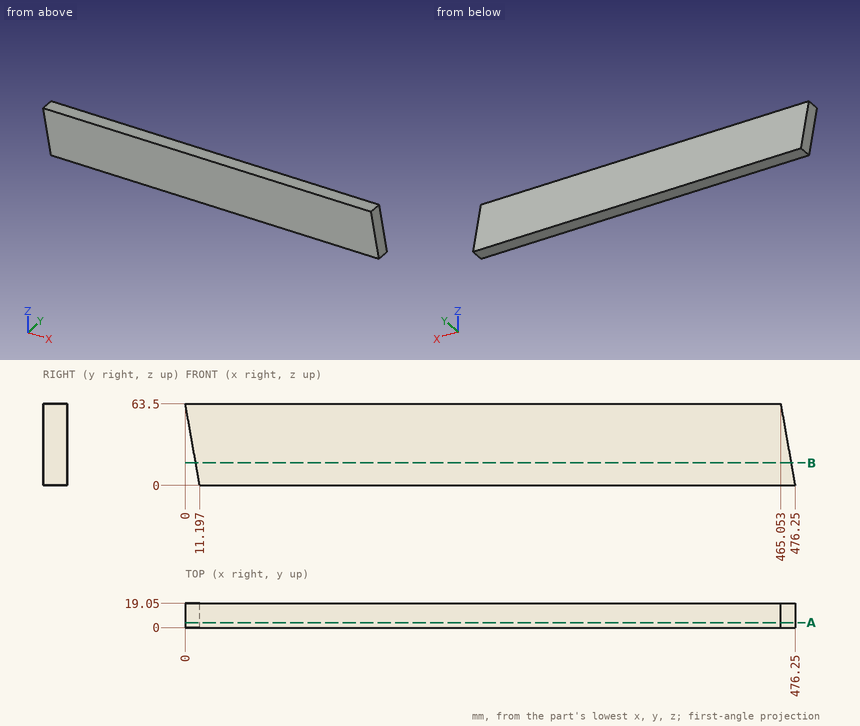
Answer from the drawing. Dimensions are ordinates in mm from the lowest x, y and z of the part. Round coordinates to 2 decimals unless told otherwise and drop trailing zeros. Loops run counter-clockwise (first coordinate to the right, second up) from the corner with the lowest first, then second, coordinate; pieces in that order, holes last.
(1) Each of these flat-tipped pins is pushed along its axis until it touches: P1, Ø3, axis at y = 3.5, z = 15.5, coming from the +X side; P2, Ø5, axis at x = 154.5, z = 34, coming from the -Y side; P3, Ø4, axis at y = 12.5, z = 14.5, coming from the +X side; P4, Ø5, axis at y = 10.5, z = 7.5, coming from the -X side. Where does it stop, or does it pass through?
Computed values:
P1: stops at x = 473.78
P2: stops at y = 0
P3: stops at x = 474.05
P4: stops at x = 9.43
(2) The part is cut by section B-B, the plane z = 17.5. Give the vertices of the cut face in (x, y).
Computed values:
outline: (8.11, 0) - (473.16, 0) - (473.16, 19.05) - (8.11, 19.05) - close
(3) The part is cut by section A-A, the plane y = 4. Give the vertices of the cut face in (x, z), and give its area (3 significant figures).
Computed values:
outline: (0, 63.5) - (11.2, 0) - (476.25, 0) - (465.05, 63.5) - close
area: 29,500 mm2
(4) Find the intervals of material crossed by L1, parallel to X at y = 14, z = 58.5 (1 decimal); L2, parallel to X at y = 9.25, z = 43 (1 decimal), in increasing order.
Computed values:
L1: x = 0.9 to 465.9
L2: x = 3.6 to 468.7
